Here's how the part is built. I have some questions about the finished solid (model axes, mm). A direction names the side the tool comes from. Round coordinates to 2 decimals unless told otherwise and drop trailing zeros. Loops run counter-clockwise (first coordinate to the right, second up) from the corner with the lowest first, then second, coordinate; pieces in that order, holes last. Notation, with made-up numbers: M -21.5,-13 L -1.5,-13 A3 cw -1.5,-8 Z; hole C 77.25,74.25 d9. An arc over 180 degrees is marked long. Answer as a JSON object with one key per item and string values.
from build123d import *

# Parameters (mm, degrees)
SKETCH2_W           = 400
SKETCH2_H           = 8
SKETCH3_W           = 16
SKETCH3_H           = 40
BOSS_EXTRUDE1_DEPTH = 4
SKETCH5_R           = 4
CUT_EXTRUDE1_DEPTH  = 4


with BuildPart() as part:
    # Sketch2 → Revolve1 (revolve)
    with BuildSketch(Plane(origin=(0, 0, 0), x_dir=(-1, 0, 0), z_dir=(0, 1, 0))):
        with Locations((0, -4)):
            Rectangle(SKETCH2_W, SKETCH2_H)
    revolve(axis=Axis((200, 0, 0), (-1, 0, 0)))

    # Sketch3 → Boss-Extrude1 (add)
    with BuildSketch(Plane.YZ.offset(200)):
        with Locations((0, 12)):
            Rectangle(SKETCH3_W, SKETCH3_H)
    extrude(amount=BOSS_EXTRUDE1_DEPTH)

    # Sketch5 → Cut-Extrude1 (cut)
    with BuildSketch(Plane(origin=(200, 0, 0), x_dir=(0, -1, 0), z_dir=(-1, 0, 0))):
        with Locations(Location((0, 25, 0), (0, 0, 90))):
            Circle(SKETCH5_R)
    extrude(amount=-CUT_EXTRUDE1_DEPTH, mode=Mode.SUBTRACT)


solid = part.part
Item 1: Please list where these lines run through material, in increasing order: probe 1 along Y at (x, z) = (202, 25); probe 2 along Z at (x, y) = (-158, 0.5); probe 3 along X at (y, z) = (5, 7). Write a range as from..to.
Resolved:
{"probe 1": "-8..-4, 4..8", "probe 2": "-7.98..7.98", "probe 3": "200..204"}
Item 2: On a 3-axis mill with a long thin cutter (end or side, diameter ignored), from which of +Z, -Z, +X, -X, +Y, -Y can I reach the whole of each face in a straight line? I mean faces 1 (the face through (200, -6, -6)), 2 (the face through (204, 0, 12)). Say none if no direction works.
Resolved:
{"face 1": "-Z, -X, -Y", "face 2": "+Z, -Z, +X, +Y, -Y"}
Item 3: I want a section at A-A, the plane z = 25. Please give me the cut outline in (x, y), then the cut area to 3 significant figures.
Resolved:
{"outline": "M 200,-8 L 204,-8 L 204,-4 L 200,-4 Z; M 200,4 L 204,4 L 204,8 L 200,8 Z", "area": "32.0 mm²"}
Item 4: I'm going to push flat-ended pins straight in: pin 1 Ø5 at (x, y) = (134.5, 6.5) entering from -Z; pin 2 Ø4 at (y, z) = (0, 22.5) entering from -X. Where does each tip first touch, or does it pass through?
Resolved:
{"pin 1": "z = -6.93", "pin 2": "x = 200"}
Item 5: If we mould it in two halves opening along Y, with no side actions, what happens to faces 3 (the face through (-2.8, 7.81, 1.73)), 4 (the face through (202, -2.4, 21.8)), 5 (the face through (200, 6, -6))? For each: pulls with the +Y half, pulls with the -Y half, needs draft (parallel to the pull), parting line crosses it, or undercut.
Resolved:
{"face 3": "parting line crosses it", "face 4": "undercut", "face 5": "needs draft"}
Item 6: I want a section at B-B, the plane x = -170.5. Please give me the cut outline in (y, z).
Resolved:
{"outline": "C 0,0 d16"}
